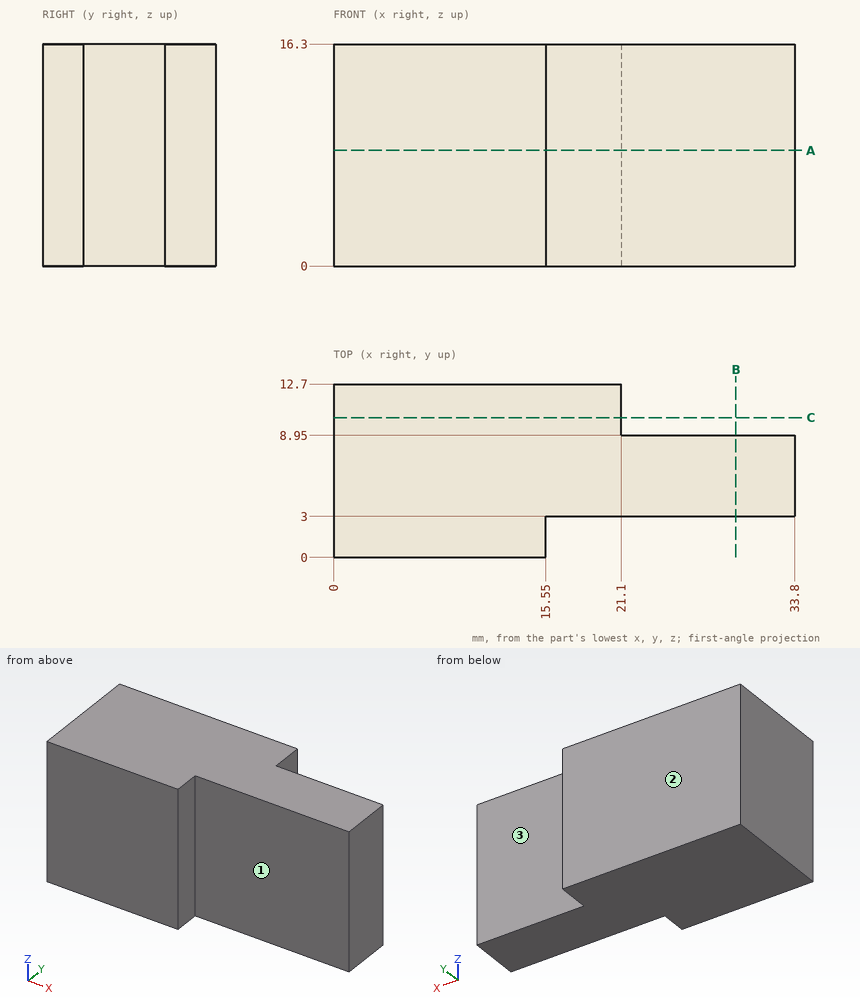
Could you check a few things on this drawing? It's one solid part, dimensions in mm from its lowest x, y, z. A direction names the side the tool comes from. Round coordinates to 2 decimals unless told otherwise and drop trailing zeros. Order: outer loops, then holes, each group sorted by start corner. A loop starts at its lowest first (then second) coordinate and runs counter-clockwise, first axis right, second up.
Q1. Imagine slicing it at B-B, the plane x = 29.5. List the corners of the cut face in (y, z) for me, then the cut area to 3 significant figures.
Geometry says:
outline: (3, 0) - (8.95, 0) - (8.95, 16.3) - (3, 16.3) - close
area: 97.0 mm2
Q2. Imagine slicing it at C-C, the plane y = 10.25. List the corners of the cut face in (x, z) for me.
Geometry says:
outline: (0, 0) - (21.1, 0) - (21.1, 16.3) - (0, 16.3) - close
Q3. Which directions (+Z, -Z, +X, -X, +Y, -Y) give clear straight access to the entire face, cutting with the end or side of a thin tool? Please do the marked faces 1, 2 and 3.
Geometry says:
face 1: +Z, -Z, +X, -Y
face 2: +Z, -Z, +X, -X, +Y
face 3: +Z, -Z, +X, +Y
Q4. Please list where these lines run through material, in increasing order: probe 1 along X at (y, z) = (11.75, 2.75); probe 2 along Y at (x, z) = (23.5, 13.25); probe 3 along Y at (x, z) = (18.5, 3).
Geometry says:
probe 1: x = 0 to 21.1
probe 2: y = 3 to 8.95
probe 3: y = 3 to 12.7
Q5. I'm going to push flat-ended pins straight in: P1, Ø3, axis at y = 11.5, z = 11, coming from the +X side; P2, Ø2.5, axis at y = 1.5, z = 6, coming from the +X side; P3, Ø6, axis at x = 27.5, z = 9.5, coming from the -Y side. Where does each tip first touch, or does it pass through?
Geometry says:
P1: stops at x = 21.1
P2: stops at x = 15.55
P3: stops at y = 3
Q6. Imagine slicing it at A-A, the plane z = 8.5. List the corners of the cut face in (x, y) for me.
Geometry says:
outline: (0, 0) - (15.55, 0) - (15.55, 3) - (33.8, 3) - (33.8, 8.95) - (21.1, 8.95) - (21.1, 12.7) - (0, 12.7) - close
